from build123d import *
from OCP.BRepFilletAPI import BRepFilletAPI_MakeChamfer

# Parameters (mm, degrees)
SKETCH1_W                             = 38.1
SKETCH1_H                             = 31.75
BOSS_EXTRUDE1_DEPTH                   = 10
CUT_EXTRUDE1_REACH                    = 28.738
SKETCH2_W                             = 34.1
SKETCH2_H                             = 25.4
F_1_8_0_125_DIAMETER_HOLE1_AT_2_COUNT = 2
F_1_8_0_125_DIAMETER_HOLE1_AT_2_PITCH = 12.7
DRAFT1_ANGLE                          = 3
CUT_EXTRUDE2_DEPTH                    = 28.969652512
CUT_EXTRUDE3_DEPTH                    = 35.177500808
FILLET2_R                             = 3.175
CHAMFER1_SIZE                         = 0.5
CHAMFER2_SIZE                         = 0.5
CHAMFER2_SIZE2                        = 0.528377251


with BuildPart() as part:
    # Sketch1 → Boss-Extrude1 (new body)
    with BuildSketch(Plane(origin=(0, 0, 0), x_dir=(1, 0, 0), z_dir=(0, 1, 0))):
        Rectangle(SKETCH1_W, SKETCH1_H)
    extrude(amount=BOSS_EXTRUDE1_DEPTH)

    # Sketch2 → Cut-Extrude1 (cut, up to next)
    with BuildSketch(Plane(origin=(0, 10, 0), x_dir=(1, 0, 0), z_dir=(0, 1, 0)), mode=Mode.PRIVATE) as cut_extrude1_sk1:
        with Locations((2, 3.175)):
            Rectangle(SKETCH2_W, SKETCH2_H)
    cut_extrude1_tool1 = extrude(cut_extrude1_sk1.sketch, amount=-CUT_EXTRUDE1_REACH, mode=Mode.PRIVATE) & part.part
    add(cut_extrude1_tool1.solids().sort_by_distance((2, 10, -3.175))[0], mode=Mode.SUBTRACT)

    # Sketch3 → 1/8 (0.125) Diameter Hole1 (revolve, cut)
    with BuildSketch(Plane(origin=(-19.05, 5, -9.525), x_dir=(0, 0, 1), z_dir=(0, 1, 0))):
        Polygon((0, 0), (0, 4), (2.2225, 4), (1.5875, 3.365), (1.5875, 0.635), (2.2225, 0), align=None)
    f_1_8_0_125_diameter_hole1 = revolve(axis=Axis((-25.4, 5, -9.525), (1, 0, 0)), mode=Mode.SUBTRACT)

    # 1/8 (0.125) Diameter Hole1 at 2: 1/8 (0.125) Diameter Hole1 ×2
    with Locations(*[(0, 0, i * F_1_8_0_125_DIAMETER_HOLE1_AT_2_PITCH) for i in range(1, F_1_8_0_125_DIAMETER_HOLE1_AT_2_COUNT)]):
        add(f_1_8_0_125_diameter_hole1, mode=Mode.SUBTRACT)

    # Draft1
    draft1_faces = [part.faces().sort_by_distance(p)[0] for p in [
        (0, 5, 15.875),
    ]]
    draft(draft1_faces, Plane(origin=(-19.05, 10, 15.875), x_dir=(0, 0, -1), z_dir=(-1, 0, 0)), DRAFT1_ANGLE)

    # Sketch7 → Cut-Extrude2 (cut, through all)
    with BuildSketch(Plane(origin=(0, 10, 0), x_dir=(1, 0, 0), z_dir=(0, 1, 0))):
        Polygon((-15.05, -9.525), (19.05, -9.525), (19.05, -11.312105274), align=None)
    extrude(amount=-CUT_EXTRUDE2_DEPTH, mode=Mode.SUBTRACT)

    # Sketch8 → Cut-Extrude3 (cut, through all)
    with BuildSketch(Plane(origin=(-0.539039544, 0, 10.285487213), x_dir=(-0.9986295347545739, 0, -0.05233595624294398), z_dir=(0.05233595624294399, 0, -0.998629534754574))):
        with BuildLine():
            Line((-6.869125485, 7.5), (1.130874515, 7.5))
            ThreePointArc((1.130874515, 7.5), (3.630874515, 5), (1.130874515, 2.5))
            Line((1.130874515, 2.5), (-6.869125485, 2.5))
            ThreePointArc((-6.869125485, 2.5), (-9.369125485, 5), (-6.869125485, 7.5))
        make_face()
    extrude(amount=-CUT_EXTRUDE3_DEPTH, mode=Mode.SUBTRACT)

    # Fillet2
    fillet2_edges = [part.edges().sort_by_distance(p)[0] for p in [
        (-15.05, 5, 9.525),
    ]]
    fillet(fillet2_edges, radius=FILLET2_R)

    # Chamfer1
    chamfer1_edges = [part.edges().sort_by_distance(p)[0] for p in [
        (8.817245881, 5, 10.775829354),
        (2.326153905, 2.5, 10.435645639),
        (-4.164938071, 5, 10.095461923),
        (2.326153905, 7.5, 10.435645639),
    ]]
    chamfer(chamfer1_edges, length=CHAMFER1_SIZE)

    # Chamfer2: one chamfer whose edges measure the first distance from different faces: ONE call of the kernel's chamfer builder (chamfer() names one face for all edges)
    chamfer2_edges_1 = [part.edges().sort_by_distance(p)[0] for p in [
        (-15.05, 0, -4.68148125),
        (-15.05, 5, -15.875),
        (-15.05, 10, -4.68148125),
        (3.504416669, 10, 10.497395774),
        (3.504416669, 0, 10.497395774),
        (-14.178063628, 10, 8.697563279),
        (-14.178063628, 0, 8.697563279),
    ]]
    chamfer2_edges_2 = [part.edges().sort_by_distance(p)[0] for p in [
        (19.05, 5, 11.312105274),
    ]]
    chamfer2_side_2 = [part.faces().sort_by_distance(p)[0] for p in [
        (9.643116423, 5, 10.819111395),
    ]]
    chamfer2 = BRepFilletAPI_MakeChamfer(part.part.solid().wrapped)
    for e in chamfer2_edges_1:
        chamfer2.Add(CHAMFER2_SIZE, e.wrapped)
    for e in chamfer2_edges_2:
        chamfer2.Add(CHAMFER2_SIZE, CHAMFER2_SIZE2, e.wrapped, chamfer2_side_2[0].wrapped)  # the first distance lies on this face
    add(Compound.cast(chamfer2.Shape()), mode=Mode.REPLACE)


solid = part.part
Can you work these out from the model? Positions are in its coordinate system, mm. A direction names the side the tool comes from. Coordinates: 2 decimals unless noted, no trailing zeros. Order: outer loops, then holes, each group sorted by start corner. A loop starts at its lowest first (then second) coordinate and runs counter-clockwise, first axis right, second up. Notation, with made-up numbers: (6.25, -8) -> (45.25, -8) arc R26 ccw to (45.25, 30) -> close; hole circle Ø11 at (39.5, 50). An arc over 180 degrees is marked (long way). Use one line per item in the form item = value.
Q1. Imagine slicing it at C-C, the plane x = 11. List the corners of the cut face in (y, z) for me, then the cut area to 3 significant figures.
From the geometry:
outline = (0, 11.39) -> (0.5, 10.89) -> (9.5, 10.89) -> (10, 11.39) -> (10, 17.45) -> (0, 17.45) -> close
area = 65.3 mm²
Q2. Imagine slicing it at A-A, the plane z = -6. List the corners of the cut face in (x, y) for me.
From the geometry:
outline = (-19.05, 0) -> (-15.55, 0) -> (-15.05, 0.5) -> (-15.05, 9.5) -> (-15.55, 10) -> (-19.05, 10) -> close
Q3. Will these pins go through, and if not, where does the flat tip stop? P1, Ø4, axis at x = 4, y = 3.5, coming from the +Z side; P2, Ø3, axis at x = 13, y = 5, coming from the -Z side; P3, Ø3, axis at y = 2, z = -10, coming from the +X side.
From the geometry:
P1 = 17.17
P2 = 10.92
P3 = -15.05
Q4. We'd pull the mould along Y, two halves only. Please class faces 1 (the face through (2.257, 2.253, 10.686)), 2 (the face through (-14.3, 0.36, 8.77)), 3 (the face through (3.469, 9.063, 10.496)): released by +Y, released by -Y, zero draft, split by the parting line, or undercut.
From the geometry:
face_1 = undercut
face_2 = released by -Y
face_3 = zero draft
Q5. I need wall thicknesses on L1, parallel to Z at x = -15.5, y = 5.5 (3 decimals); L2, parallel to Z at x = -16.95, y = 5 (1 decimal); L3, parallel to X at y = 3.75, z = -3. Which ranges of each line are inside material? Lowest first, please.
From the geometry:
L1 = -15.825 to -11.226, -7.824 to 1.474, 4.876 to 16.061
L2 = -15.9 to -11.1, -7.9 to 1.6, 4.8 to 16
L3 = -19.05 to -15.05
Q6. Which directions (+Z, -Z, +X, -X, +Y, -Y) give clear straight access to the entire face, cutting with the end or side of a thin tool? Please do faces 4 (the face through (2, 2.5, 14)), 5 (the face through (2.37, 7.75, 10.69)), 6 (the face through (3.274, 0.254, 10.732)).
From the geometry:
face_4 = +Z, -Z
face_5 = -Z
face_6 = -Z, +X, -Y
Q7. Imagine slicing it at B-B, the plane y = 5. Give the number of separate pieces and of enclosed holes in the cut face, then the cut area to 3 significant figures.
From the geometry:
separate_pieces = 4
enclosed_holes = 0
area = 240 mm²
